from build123d import *

# Parameters (mm, degrees)
SKETCH1_W           = 1000
SKETCH1_H           = 270
BOSS_EXTRUDE1_DEPTH = 50
FILLET1_R           = 100
FILLET2_R           = 20


with BuildPart() as part:
    # Sketch1 → Boss-Extrude1 (new body)
    with BuildSketch(Plane(origin=(0, 0, 0), x_dir=(1, 0, 0), z_dir=(0, 1, 0))):
        with Locations((-500, 135)):
            Rectangle(SKETCH1_W, SKETCH1_H)
    extrude(amount=BOSS_EXTRUDE1_DEPTH)

    # Fillet1
    fillet1_edges = [part.edges().sort_by_distance(p)[0] for p in [
        (0, 25, 0),
        (0, 25, -270),
    ]]
    fillet(fillet1_edges, radius=FILLET1_R)

    # Fillet2
    fillet2_edges = [part.edges().sort_by_distance(p)[0] for p in [
        (-550, 0, -270),
        (-550, 50, -270),
        (0, 0, -135),
        (-550, 0, 0),
        (-29.289321881, 0, -29.289321881),
        (-29.289321881, 0, -240.710678119),
        (0, 50, -135),
        (-550, 50, 0),
        (-29.289321881, 50, -29.289321881),
        (-29.289321881, 50, -240.710678119),
    ]]
    fillet(fillet2_edges, radius=FILLET2_R)


solid = part.part
Can you work these out from the model? Positions are in its coordinate system, mm. Round coordinates to 2 decimals unless told otherwise and drop trailing zeros. Loops run counter-clockwise (first coordinate to the right, second up) from the corner with the lowest first, then second, coordinate; pieces in that order, holes last. Notation, with made-up numbers: (64, 10.5) - (88, 10.5) arc R21 ccw to (88, 15.5) - close; hole circle Ø9 at (7.5, -27). An arc over 180 degrees is marked (long way). Use CSV: the item, a comma, the result in double quotes. Start each with the question number.
1) For pin 1 Ø3 at (y, z) = (13, -130) entering from +X; pin 2 Ø6 at (x, y) = (-654, 16) entering from +Z (3 decimals), each with a flat end and sliding along its axis, tell me the tip position at first contact or that it passes through.
2) If we section it at A-A on x = -642: Write out the boundary of the cut face in (y, z).
3) Please list where these lines run through material, in increasing order: probe 1 along Z at (x, y) = (-899, 32); probe 2 along Z at (x, y) = (-388.5, 31); probe 3 along X at (y, z) = (22, -170.5). Write a range as [from, to].
4) If we section it at B-B on y = 11.5: Write out the boundary of the cut face in (x, z).
Geometry results:
1,pin 1,"stops at x = -0.77"
1,pin 2,"stops at z = -0.025"
2,outline,"(0, -250) arc R20 ccw to (20, -270) - (30, -270) arc R20 ccw to (50, -250) - (50, -20) arc R20 ccw to (30, 0) - (20, 0) arc R20 ccw to (0, -20) - close"
3,probe 1,"z = [-269.9, -0.1]"
3,probe 2,"z = [-269.97, -0.03]"
3,probe 3,"x = [-1000, 0]"
4,outline,"(-1000, -268.1) - (-100, -268.1) arc R98.1 ccw to (-1.9, -170) - (-1.9, -100) arc R98.1 ccw to (-100, -1.9) - (-1000, -1.9) - close"
